Autodesk Inventor part; units mm, degrees
ref_plane "YZ Plane" through (0, 0, 0) normal (1, 0, 0) x (0, 1, 0)
ref_plane "XZ Plane" through (0, 0, 0) normal (0, 1, 0) x (-1, 0, 0)
ref_plane "XY Plane" through (0, 0, 0) normal (0, 0, 1) x (1, 0, 0)
sketch "Sketch7" plane through (0, 0, 0) normal (0, 0, 1) x (1, 0, 0)
  line L0 (-5, 6.5) -> (5, 6.5)
  line L1 (5, 6.5) -> (5, -6.5)
  line L2 (5, -6.5) -> (-5, -6.5)
  line L3 (-5, -6.5) -> (-5, 6.5)
  line L4 (0, 6.5) -> (0, -6.5)
  line L5 (-5, 0) -> (5, 0)
  point P0 (0, 0)
  point P1 (0, 0)
  dimension "d14" = 10
  dimension "d15" = 13
extrude "Extrusion4" add sketch "Sketch7" along normal blind 10
sketch "Sketch8" plane through (5, -6.5, 0) normal (1, 0, 0) x (0, 0, -1)
  line L0 (0, 13) -> (-10, 13)
  line L1 (-5, 13) -> (-5, 0)
  line L2 (0, 0) -> (-10, 0)
  line L3 (0, 6.5) -> (-10, 6.5)
  line L4 (-10, 13) -> (-10, 0)
  line L5 (0, 0) -> (-10, 0)
  circle A0 centre (-5, 3.25) radius 1.625
  dimension "d18" = 3.25
  dimension "d27" = 3.25
extrude "Extrusion5" cut sketch "Sketch8" against normal through all contours A0 L1 | L1 A0
sketch "Sketch9" plane through (0, 0, 10) normal (0, 0, 1) x (1, 0, 0)
  line L0 (-5, 6.5) -> (-5, -6.5)
  line L1 (-5, 0) -> (5, 0)
  line L2 (5, -6.5) -> (5, 6.5)
  line L3 (0, 0) -> (0, 1.625)
  line L4 (5, 6.5) -> (-5, 6.5)
  circle A0 centre (0, 3.25) radius 1.625
  dimension "d22" = 3.25
  dimension "d28" = 3.25
extrude "Extrusion6" cut sketch "Sketch9" against normal through all contours A0
fillet "Fillet2" radius 2 4 edges at (5, 6.5, 5) (-5, 6.5, 5) (0, -6.5, 10) (0, -6.5, 0)
properties part number "CardanJoint"
Can you work these out from the model? Positions are in its coordinate system, mm. Coordinates: 2 decimals unless noted, no trailing zeros. Write each loop counter-clockwise with the first axis right and the second up, starting at its lowest first coordinate (ties: lowest second). Pieces come first, ordered by that corner, then holes. Notation, with made-up numbers: (68.5, 66.5) -> (74.5, 66.5) arc R23 ccw to (74.5, 100.5) -> close; hole circle Ø1 at (-36, 47). An arc over 180 degrees is marked (long way). Answer as CSV lines item,"result".
1) If we section it at D-D on x = -2.25: Please give me the cut outline in (y, z) (3 decimals), then the cut area to 3 significant figures.
Check result:
outline,"(-6.5, 2) arc R2 ccw to (-4.5, 0) -> (6.5, 0) -> (6.5, 10) -> (-4.5, 10) arc R2 ccw to (-6.5, 8) -> close; hole circle Ø3.25 at (-3.25, 5)"
area,"120 mm²"
2) If we section it at C-C on x = 0.75: Please give me the cut outline in (y, z) (3 decimals).
Check result:
outline,"(-6.5, 2) arc R2 ccw to (-4.5, 0) -> (1.808, 0) -> (1.808, 10) -> (-4.5, 10) arc R2 ccw to (-6.5, 8) -> close; (4.692, 0) -> (6.5, 0) -> (6.5, 10) -> (4.692, 10) -> close; hole circle Ø3.25 at (-3.25, 5)"
3) If we section it at B-B on y = 3.25: Please give me the cut outline in (x, z) (3 decimals).
Check result:
outline,"(-5, 0) -> (-1.625, 0) -> (-1.625, 10) -> (-5, 10) -> close; (1.625, 0) -> (5, 0) -> (5, 10) -> (1.625, 10) -> close"
4) Will this pin go through, and if not, where does the flat tip stop? P1, Ø3, axis at y = -3.25, z = 5, coming from the -X side.
Check result:
P1,"through"
5) If we section it at A-A on z = 5: Please give me the cut outline in (x, y) (3 decimals).
Check result:
outline,"(-5, -6.5) -> (5, -6.5) -> (5, -4.875) -> (-5, -4.875) -> close; (-5, -1.625) -> (5, -1.625) -> (5, 4.5) arc R2 ccw to (3, 6.5) -> (-3, 6.5) arc R2 ccw to (-5, 4.5) -> close; hole circle Ø3.25 at (0, 3.25)"
6) If we mould it in two halves opening along Y, with no side actions, what happens to faces 1 (the flat face through (5, -1, 5)), 2 (the cylindrical face through (-4.4, 5.93, 5.07)), 3 (the cylindrical face through (0.07, -3.179, 6.623))? For each: +Y half, -Y half, draft (parallel to the pull), parting line (faces both ways), or undercut.
Check result:
face 1,"draft"
face 2,"+Y half"
face 3,"undercut"
7) If I drill on line 1 (Y direction, x = 0, z = 7.75) (3 decimals); line 2 (Y direction, x = 0, z = 5.75) (3 decimals); line 3 (Y direction, x = 1, z = 5.5), over which ranges is the centre line in solid material (lowest first)? Write a range as from..to.
Check result:
line 1,"-6.5..1.625, 4.875..6.5"
line 2,"-6.5..-4.692, -1.808..1.625, 4.875..6.5"
line 3,"-6.5..-4.8, -1.7..1.97, 4.53..6.5"
